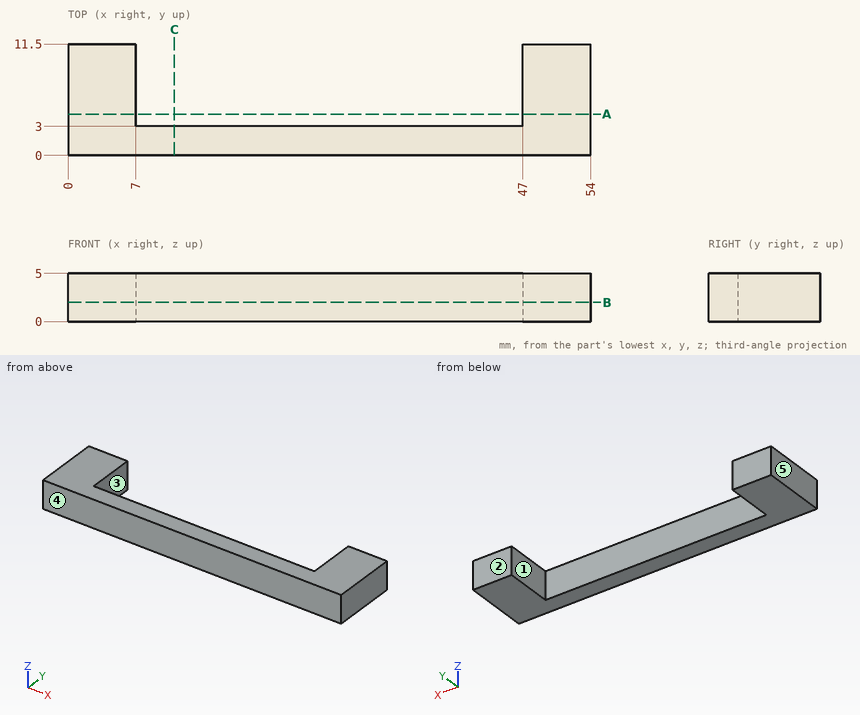
Geometry check sheet. Reference: drawing and pictorial views, mm from the part's lowest x, y, z. A direction names the side the tool comes from. Give positions to 0.01 mm unless a question says otherwise; leave off trailing zeros. Order: outer loops, then holes, each group sorted by start corner. A loop starts at its lowest first (then second) coordinate and runs counter-clockwise, first axis right, second up. Notation, with made-up numbers: (-12.5, -2) - (-4.5, -2) arc R10 ccw to (-4.5, 4) - close; hole circle Ø11 at (45, 67.25). An arc over 180 degrees is marked (long way). Use one line per item in the form item = value.
1) Depth check by flat-ended pin: pin 1 Ø1.5 at (x, z) = (32, 1.5) entering from +Y. Enter the tip coordinate at first touch or a pass-through.
Working result:
pin_1 = 3
2) Material ranges on probe 1 along X at (y, z) = (7.25, 3.85); probe 2 along Y at (x, z) = (38, 1.7), recorded low to high. Write a range as from..to.
Working result:
probe_1 = 0..7, 47..54
probe_2 = 0..3
3) Sectioned sample at A-A (y = 4.25). Record the boundary of the cut face in (x, z), and give its area (3 significant figures).
Working result:
outline = (0, 0) - (7, 0) - (7, 5) - (0, 5) - close; (47, 0) - (54, 0) - (54, 5) - (47, 5) - close
area = 70.0 mm^2
4) Sectioned sample at B-B (z = 2). Record the boundary of the cut face in (x, y).
Working result:
outline = (0, 0) - (54, 0) - (54, 11.5) - (47, 11.5) - (47, 3) - (7, 3) - (7, 11.5) - (0, 11.5) - close
5) Draft check along X on the marked faces 3, 4 and 5. Enter one of: released by +X, released by -X, zero draft, split by the parting line, or undercut.
Working result:
face_3 = undercut
face_4 = zero draft
face_5 = released by -X
6) Access from +Z, -Z, +X, -X, +Y, -Y to the whole of each face (thin tool, end or side, straight path). Record for the marked faces 1 and 2.
Working result:
face_1 = +Z, -Z, +Y
face_2 = +Z, -Z, +X, -X, +Y
7) Sectioned sample at C-C (x = 11). Record the boundary of the cut face in (y, z), and give its area (3 significant figures).
Working result:
outline = (0, 0) - (3, 0) - (3, 5) - (0, 5) - close
area = 15.0 mm^2
